Autodesk Inventor part; units mm, degrees
ref_plane "YZ Plane" through (0, 0, 0) normal (1, 0, 0) x (0, 1, 0)
ref_plane "XZ Plane" through (0, 0, 0) normal (0, 1, 0) x (-1, 0, 0)
ref_plane "XY Plane" through (0, 0, 0) normal (0, 0, 1) x (1, 0, 0)
sketch "スケッチ1" plane through (0, 0, 0) normal (0, 1, 0) x (-1, 0, 0)
  point P0 (0, 0)
sketch "スケッチ2" plane through (0, 0, 0) normal (0, 0, 1) x (1, 0, 0)
  circle A0 centre (0, 0) radius 3.5
  circle A1 centre (0, 0) radius 7.5
  line L0 (0, 0) -> (0, -152.95)
  circle A2 centre (0, -152.95) radius 4
  circle A3 centre (0, -152.95) radius 7.5
  line L1 (7.5, -152.95) -> (7.5, 0)
  line L2 (-7.5, 0) -> (-7.5, -152.95)
  dimension "d0" = 7
  dimension "d1" = 15
  dimension "d2" = 152.95
  dimension "d3" = 8
  dimension "d4" = 15
extrude "押し出し1" add sketch "スケッチ2" along normal blind 4
sketch "スケッチ4" plane through (0, 0, 4) normal (0, 0, 1) x (1, 0, 0)
  arc A0 (7.5, 0) -> (-7.5, 0) centre (0, 0) ccw
  circle A1 centre (0, 0) radius 4.25
  circle A2 centre (0, -152.95) radius 4
  circle A3 centre (0, -152.95) radius 4.75
  dimension "d10" = 8.5
  dimension "d11" = 9.5
extrude "押し出し3" cut sketch "スケッチ4" against normal blind 2
properties part number "motor_holder_top"
Verification items for the finished model (mm, model axes). A direction names the side the tool comes from. Round coordinates to 2 decimals unless told otherwise and drop trailing zeros. Write each loop counter-clockwise with the first axis right and the second up, starting at its lowest first coordinate (ties: lowest second). Pieces come first, ordered by that corner, then holes. Notation, with made-up numbers: (52, 11) -> (82, 11) arc R23 ccw to (82, 38) -> close; hole circle Ø11 at (88, -9.75). An arc over 180 degrees is marked (long way). Write each question's results on one line, items separated by ' | '. Start each with the question number.
1. Draft check along Y on faces 1 (the cylindrical face through (0.16, -160.45, 1.97)), 2 (the flat face through (0, -75, 0)), 3 (the cylindrical face through (3.233, 1.341, 0.986)). Enter one of: +Y half, -Y half, draft (parallel to the pull), parting line (faces both ways), or undercut.
2. Depth check by flat-ended pin: P1, Ø8, axis at x = 0, y = 0, coming from the +Z side; P2, Ø7.5, axis at x = 0, y = 0, coming from the -Z side; P3, Ø2, axis at x = 2, z = 2.5, coming from the +Y side. Enter the tip coordinate at first touch or a pass-through.
3. Material ranges on probe 1 along Y at (x, z) = (0, 2.6); probe 2 along Y at (x, z) = (0, 0.7); probe 3 along X at (y, z) = (0, 0.65), recorded low to high. Write a range as from..to.
4. Set-up check for faces 4 (the cylindrical face through (-0.867, -149.045, 0.986)), 5 (the cylindrical face through (-0.62, -148.24, 3.01)): record each of +Z, -Z, +X, -X, +Y, -Y from which the full face is reachable in a straight line by a thin tool's end or side.
5. Cross-section at A-A (x = 0). Enter the section's corners in (y, z).
Solutions:
1) face 1: -Y half | face 2: draft | face 3: undercut
2) P1: stops at z = 2 | P2: stops at z = 0 | P3: stops at y = 7.43
3) probe 1: y = -160.45..-157.7, -148.2..-4.25, 4.25..7.5 | probe 2: y = -160.45..-156.95, -148.95..-3.5, 3.5..7.5 | probe 3: x = -7.5..-3.5, 3.5..7.5
4) face 4: +Z, -Z | face 5: +Z
5) outline: (-160.45, 0) -> (-156.95, 0) -> (-156.95, 2) -> (-157.7, 2) -> (-157.7, 4) -> (-160.45, 4) -> close; (-148.95, 0) -> (-3.5, 0) -> (-3.5, 2) -> (-4.25, 2) -> (-4.25, 4) -> (-148.2, 4) -> (-148.2, 2) -> (-148.95, 2) -> close; (3.5, 0) -> (7.5, 0) -> (7.5, 4) -> (4.25, 4) -> (4.25, 2) -> (3.5, 2) -> close
